Autodesk Inventor part; units mm, degrees
ref_plane "Work Plane1" through (200, 2, 1.4361) normal (0, 1, 0) x (1, 0, 0)
ref_plane "YZ Plane" through (0, 0, 0) normal (1, 0, 0) x (0, 1, 0)
ref_plane "XZ Plane" through (0, 0, 0) normal (0, 1, 0) x (-1, 0, 0)
sketch "Sketch1" plane through (0, 0, 0) normal (0, 1, 0) x (-1, 0, 0)
  line L0 (0, 0) -> (-250, 0)
  line L1 (-250, 0) -> (-250, -30)
  line L2 (-250, -30) -> (0, -30)
  line L3 (0, -30) -> (0, 0)
  dimension "d0" = 250
  dimension "d1" = 30
extrude "Extrusion1" add sketch "Sketch1" along normal blind 2
sketch "Sketch2" plane through (250, 0, 0) normal (1, 0, 0) x (0, 0, -1)
  circle A0 centre (0, 3) radius 1.25
  circle A1 centre (0, 3) radius 1.75
  point P0 (0, 0)
  dimension "d4" = 2.5
  dimension "d5" = 3
  dimension "d6" = 3.5
extrude "Extrusion2" add sketch "Sketch2" against normal blind 250
extrude "Extrusion3" cut sketch "Sketch2" against normal blind 250 contours A0
sketch "Sketch3" plane through (250, 0, -30) normal (0, 0, -1) x (-1, 0, 0)
  line L0 (50, 4.75) -> (100, 4.75)
  line L1 (100, 4.75) -> (100, 2)
  line L2 (100, 2) -> (50, 2)
  line L3 (50, 2) -> (50, 4.75)
  line L4 (150, 4.75) -> (200, 4.75)
  line L5 (200, 4.75) -> (200, 2)
  line L6 (200, 2) -> (150, 2)
  line L7 (150, 2) -> (150, 4.75)
  point P0 (0, 2)
  point P1 (75, 2)
  point P2 (175, 2)
  point P3 (250, 2)
  dimension "d38" = 50
  dimension "d39" = 2.75
  dimension "d40" = 50
  dimension "d41" = 2.75
  dimension "d42" = 50
  dimension "d43" = 50
ref_plane "Work Plane1" through (200, 2, 1.4361) normal (0, 1, 0) x (1, 0, 0)
sketch "Sketch5" plane through (0, 2, 0) normal (0, 1, 0) x (1, 0, 0)
  line L0 (100, 1.75) -> (100, -1.75)
  line L1 (0, 0) -> (50, 0)
  point P0 (25, 10)
  point P1 (65, 20)
  point P2 (105, 10)
  point P3 (145, 20)
  point P4 (185, 10)
  point P5 (225, 20)
  point P6 (100, 0)
  point P7 (100, 1.4361)
  dimension "d23" = 40
  dimension "d24" = 5
  dimension "d25" = 40
  dimension "d26" = 40
  dimension "d27" = 40
  dimension "d28" = 40
  dimension "d29" = 10
  dimension "d30" = 10
hole "Hole1" at (25, 2, -10) at (65, 2, -20) at (105, 2, -10) at (145, 2, -20) at (185, 2, -10) at (225, 2, -20) direction (0, -1, 0) diameter 3 end through all countersink diameter 5 countersink angle 90
extrude "Extrusion6" cut sketch "Sketch3" against normal through all
sketch "Sketch6" plane through (150, 2, 1.4361) normal (0, 1, 0) x (1, 0, 0)
  line L0 (-50, 0) -> (-100, 0)
  line L1 (-50, 2.6861) -> (-50, 0.1861)
  line L2 (-100, 0) -> (-50, 0)
  line L3 (-50, 0) -> (-50, 1.4361)
  line L4 (-50, 1.4361) -> (-100, 1.4361)
  line L5 (-100, 1.4361) -> (-100, 0)
  line L6 (0, 0.6861) -> (0, 0)
  line L7 (50, 2.6861) -> (50, 0.1861)
  line L8 (0, 0) -> (50, 0)
  line L9 (50, 0) -> (50, 1.4361)
  line L10 (50, 1.4361) -> (0, 1.4361)
  line L11 (0, 1.4361) -> (0, 0)
  point P0 (-150, 1.4361)
  point P1 (-50, 0.6861)
  point P2 (-50, 2.1861)
  point P3 (50, 0.6861)
  point P4 (50, 2.1861)
extrude "Extrusion7" cut sketch "Sketch6" against normal through all
equation "\"d40\" = d38"
equation "\"d43\" = d38"
properties part number "Hinge 2 of 2" material "Steel"
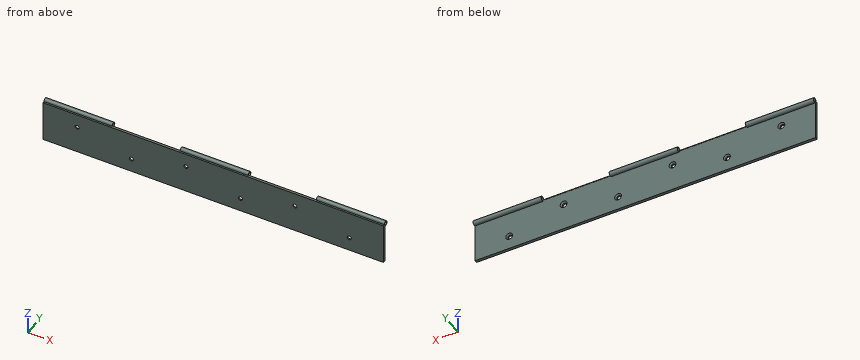
Here's how the part is built. I have some questions about the finished solid (model axes, mm). Give positions to 0.01 mm unless a question says otherwise; leave off trailing zeros. Write each loop counter-clockwise with the first axis right and the second up, starting at its lowest first coordinate (ties: lowest second). Pieces come first, ordered by that corner, then holes. Notation, with made-up numbers: (41.25, 9.5) -> (52.25, 9.5) arc R20 ccw to (52.25, 35.5) -> close; hole circle Ø5 at (55.25, -13). An arc over 180 degrees is marked (long way). Use one line per item in the form item = value.
1) I'm going to push flat-ended pins straight in: pin 1 (1 mm diameter, centred on x = 171.5, y = 0.5, fed in from +Z); pin 2 (1 mm diameter, centred on y = 3.5, z = 0.5, fed in from -X); pin 3 (9 mm diameter, centred on x = 161.5, z = -20, fed in from +Y); pin 4 (3.5 mm diameter, centred on x = 145, z = -20, fed in from +Y). Where does each tip first touch, or does it pass through?
Verdict:
pin_1 = 0
pin_2 = through
pin_3 = 2
pin_4 = 1.25
2) Suppose I cut it at A-A (y = 3). Please give me the cut outline in (x, z).
Verdict:
outline = (0, -1.75) -> (50, -1.75) -> (50, -1.25) -> (0, -1.25) -> close; (0, 1.25) -> (50, 1.25) -> (50, 1.75) -> (0, 1.75) -> close; (100, -1.75) -> (150, -1.75) -> (150, -1.25) -> (100, -1.25) -> close; (100, 1.25) -> (150, 1.25) -> (150, 1.75) -> (100, 1.75) -> close; (200, -1.75) -> (250, -1.75) -> (250, -1.25) -> (200, -1.25) -> close; (200, 1.25) -> (250, 1.25) -> (250, 1.75) -> (200, 1.75) -> close
3) Suppose I cut it at B-B (x = 179). Please give me the cut outline in (y, z), and give its area (3 significant figures).
Verdict:
outline = (0, -30) -> (2, -30) -> (2, -0.75) arc R1.25 cw to (1.75, 0) -> (0, 0) -> close
area = 59.9 mm2
4) Suppose I cut it at C-C (x = 128.5). Please give me the cut outline in (y, z), and give its area (3 significant figures).
Verdict:
outline = (0, -30) -> (2, -30) -> (2, -1.44) arc R1.75 ccw (long way) to (1.25, 0) -> (0, 0) -> close; hole circle Ø2.5 at (3, 0)
area = 64.0 mm2
5) If I drill on L1, parallel to X at y = 0.4, z = -20; L2, parallel to Z at x = 185, y = 0.8; L3, parallel to Z at x = 125.5, y = 3, over which ranges is the centre line in solid material (lowest first)? Write a range as [from, to].
Verdict:
L1 = [0, 63.5], [66.5, 143.5], [146.5, 223.5], [226.5, 250]
L2 = [-30, -11.5], [-8.5, 0]
L3 = [-1.75, -1.25], [1.25, 1.75]
